Autodesk Inventor part; units mm, degrees
ref_plane "YZ Plane" through (0, 0, 0) normal (1, 0, 0) x (0, 1, 0)
ref_plane "XZ Plane" through (0, 0, 0) normal (0, 1, 0) x (-1, 0, 0)
ref_plane "XY Plane" through (0, 0, 0) normal (0, 0, 1) x (1, 0, 0)
sketch "Boceto1" plane through (0, 0, 0) normal (0, 1, 0) x (-1, 0, 0)
  circle A0 centre (0, 0) radius 25
  circle A1 centre (0, 0) radius 20
  line L0 (0, 0) -> (25, 0)
  line L1 (0, 0) -> (17.6777, -17.6777)
  line L2 (0, 0) -> (25, 0) construction
  line L3 (0, 0) -> (17.6777, 17.6777)
  line L4 (0, 0) -> (25, 0) construction
  line L5 (0, 0) -> (-17.6777, -17.6777)
  line L6 (0, 0) -> (-17.6777, 17.6777)
  circle A2 centre (20, 0) radius 3
  circle A3 centre (14.1421, -14.1421) radius 3
  circle A4 centre (14.1421, 14.1421) radius 3
  circle A5 centre (-14.1421, 14.1421) radius 3
  circle A6 centre (-14.1421, -14.1421) radius 3
  point P0 (16.0984, 11.8677)
  point P1 (11.8677, 16.0984)
  dimension "d0" = 50
  dimension "d1" = 40
  dimension "d2" = 45
  dimension "d3" = 45
  dimension "d4" = 6
  dimension "d5" = 6
  dimension "d6" = 6
  dimension "d7" = 6
  dimension "d8" = 6
extrude "Extrusión1" add sketch "Boceto1" along normal blind 10 contours L0 A2 A1 A4 L3 A0 | A0 L1 A3 A1 A2 L0 | L3 A4 A1 A5 L6 A0 | A0 L5 A6 A1 A3 L1 | L6 A5 A1 A6 L5 A0 | A2 L0 L3 A4 A1 | A1 A3 L1 L0 A2 | A4 L3 L6 A5 A1 | A1 A6 L5 L1 A3 | A5 L6 L5 A6 A1
thread "Rosca1"
thread "Rosca2"
thread "Rosca3"
thread "Rosca4"
sketch "Boceto3" plane through (0, 10, 0) normal (0, 1, 0) x (1, 0, 0)
  circle A0 centre (0, 0) radius 12.5
  dimension "d22" = 25
extrude "Extrusión3" add sketch "Boceto3" along normal blind 6
sketch "Boceto7" plane through (0, 0, 0) normal (0, 0, 1) x (1, 0, 0)
  line L0 (0, 0) -> (0, -15)
  line L1 (0, -15) -> (14.1421, -29.1421)
  dimension "d31" = 15
  dimension "d32" = 20
  dimension "d33" = 135
sketch "Boceto8" plane through (0, 0, 0) normal (0, -1, 0) x (1, 0, 0)
  circle A0 centre (0, 0) radius 13.9045
  dimension "d34" = 27.809
sweep "Barrido1" add profiles "Boceto8" path "Boceto7"
sketch "Boceto10" plane through (14.1421, -29.1421, 0) normal (0.7071, -0.7071, 0) x (-0.7071, -0.7071, 0)
  ellipse E0 centre (-17.6777, 0) end of major axis (-17.6777, -25) minor radius 17.6777
  circle A0 centre (0, 0) radius 13.9045
  circle A1 centre (0, 0) radius 10.9045
  point P0 (-10.6066, 0)
  dimension "d40" = 27.809
  dimension "d41" = 21.809
extrude "Extrusión7" cut sketch "Boceto10" against normal blind 14 contours A0 E0 A1 | E0 A1 A0
sketch "Boceto11" plane through (14.1421, -29.1421, 0) normal (0.7071, -0.7071, 0) x (-0.7071, -0.7071, 0)
  ellipse E0 centre (-17.6777, 0) end of major axis (-17.6777, -25) minor radius 17.6777
  circle A0 centre (0, 0) radius 3.05
  point P0 (-10.6066, 0)
  dimension "d44" = 6.1
extrude "Extrusión8" cut sketch "Boceto11" against normal blind 10 contours A0 E0 | E0 A0 picked at (-0.8572, 1.0724) picked at (0.8995, 0.9612)
properties part number "BaseH"
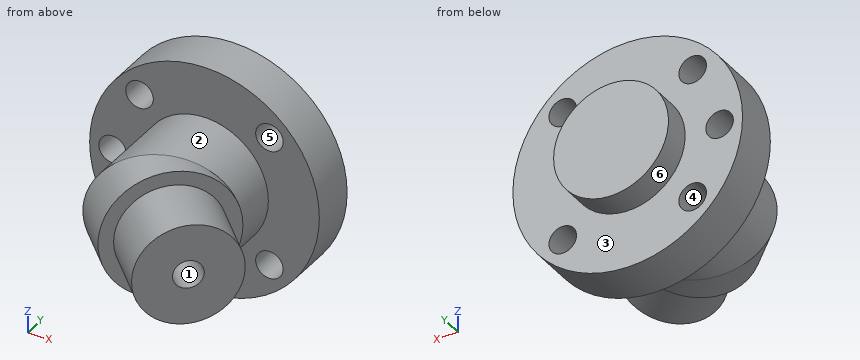
Work out the finished part from the listing and answer in its coordinate system (mm). Face numbers are marked on the shaded views. A direction names the side the tool comes from. Give positions to 0.01 mm unless a question says otherwise; leave off trailing zeros. Loops run counter-clockwise (first coordinate to the right, second up) from the corner with the lowest first, then second, coordinate; pieces in that order, holes last. Notation, with made-up numbers: (67, 25.5) -> (107, 25.5) arc R14 ccw to (107, 51.5) -> close; hole circle Ø7 at (87, 9.5). An arc over 180 degrees is marked (long way). Use a Markdown table: item, result. Add a question column.
1. For the marked faces 5 and 6, determine the directions among +Z, -Z, +X, -X, +Y, -Y from which every point of the face is accessible in a straight line to the end or side of a thin tool.
2. Section C-C on y = 2 is taken. Determine the outline of the cut face in (x, z).
3. Section D-D on z = -9.5 is taken. Determine the outline of the cut face in (x, y).
4. Find the intervals of material crossed by probe 1 along X at (y, z) = (2, 13); probe 2 along Z at (x, y) = (12, -28); probe 3 along X at (y, z) = (3, -12), in increasing order.
5. Flat-ended cylindrical pins translate along their axes: pin 1 Ø6 at (y, z) = (-13, 10) entering from -X; pin 2 Ø5.5 at (x, z) = (-14.14, -14.14) entering from -Y; pin 3 Ø12 at (y, z) = (-8, 8.5) entering from -X; pin 4 Ø3 at (x, z) = (-5, -11.5) entering from -Y. Find the tip coordinate at first contact, or state that the pin passes through.
6. Determine the mould class of the marked faces 1, 2, 3 and 4 for opening direction Z: released by +Z, released by -Z, zero draft, split by the parting line, or undercut.
7. Section A-A on x = -20 is taken. Determine the outline of the cut face in (y, z).
8. Section B-B on z = 0 is taken. Determine the outline of the cut face in (x, y).
Results below:
| question | item | result |
|---|---|---|
| 1 | face 5 | +Y, -Y |
| 1 | face 6 | +Y |
| 2 | outline | circle Ø50 at (0, 0); hole circle Ø6 at (-20, 0); hole circle Ø6 at (-14.14, -14.14); hole circle Ø6 at (-14.14, 14.14); hole circle Ø6 at (14.14, -14.14); hole circle Ø6 at (14.14, 14.14) |
| 3 | outline | (-23.12, 0) -> (-10.15, 0) -> (-10.15, -19.21) -> (-2.94, -26.42) -> (0.46, -23.03) -> (10.36, -32.93) -> (17.93, -25.36) -> (8.03, -15.46) -> (11.42, -12.06) -> (10.15, -10.79) -> (10.15, 0) -> (23.12, 0) -> (23.12, 10) -> (8.12, 10) -> (8.12, 16) -> (-8.12, 16) -> (-8.12, 10) -> (-23.12, 10) -> close |
| 4 | probe 1 | x = -21.35 to -16.92, -11.37 to 11.37, 16.92 to 21.35 |
| 4 | probe 2 | z = -10.88 to -2.97, 2.97 to 10.88 |
| 4 | probe 3 | x = -21.93 to -16.24, -12.04 to 12.04, 16.24 to 21.93 |
| 5 | pin 1 | stops at x = -12.01 |
| 5 | pin 2 | passes through |
| 5 | pin 3 | stops at x = -13.68 |
| 5 | pin 4 | stops at y = -24.12 |
| 6 | face 1 | undercut |
| 6 | face 2 | split by the parting line |
| 6 | face 3 | zero draft |
| 6 | face 4 | undercut |
| 7 | outline | (0, -15) -> (10, -15) -> (10, -3) -> (0, -3) -> close; (0, 3) -> (10, 3) -> (10, 15) -> (0, 15) -> close |
| 8 | outline | (-25, 0) -> (-23, 0) -> (-23, 10) -> (-25, 10) -> close; (-17, 0) -> (-13.9, 0) -> (-13.9, -20.76) -> (-5.59, -29.07) -> (-3.47, -26.95) -> (6.43, -36.85) -> (11.99, -31.3) -> (4.91, -24.23) -> (9.23, -19.91) -> (16.3, -26.99) -> (21.85, -21.43) -> (11.95, -11.53) -> (14.07, -9.41) -> (13.9, -9.24) -> (13.9, 0) -> (25, 0) -> (25, 10) -> (12.5, 10) -> (12.5, 16) -> (-12.5, 16) -> (-12.5, 10) -> (-17, 10) -> close |
